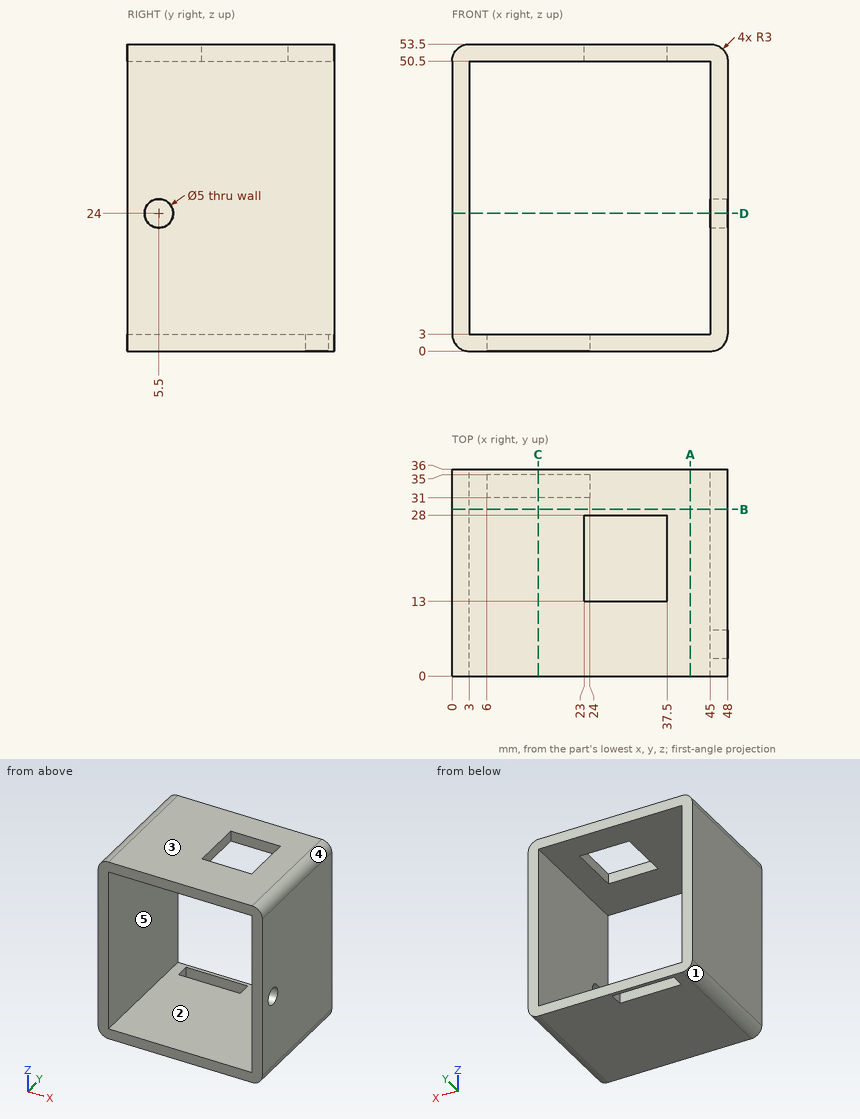
Drawing for the job (mm, zero at the part's lowest x, y, z). A direction names the side the tool comes from. Round coordinates to 2 decimals unless told otherwise and drop trailing zeros. Order: outer loops, then holes, each group sorted by start corner. A loop starts at its lowest first (then second) coordinate and runs counter-clockwise, first axis right, second up. Notation, with made-up numbers: M 56,-37 L 76,-37 A18 cw 76,-7 Z; hole C 1,18 d7. An arc over 180 degrees is marked long. Use one line per item in the form item = value.
Q1. Probe L1, parallel to X at y = 3.5, z = 5; L2, parallel to Y at x = 47.35, z = 24; L3, parallel to Z at x = 34, y = 12.5. List the from-to ranges inside material, lowest first.
Recorded:
L1 = 0 to 3, 45 to 48
L2 = 0 to 3, 8 to 36
L3 = 0 to 3, 50.5 to 53.5
Q2. Saw through at A-A on x = 41.5. Give the cut face in (y, z), then the cut area to 3 significant figures.
Recorded:
outline = M 0,0 L 36,0 L 36,3 L 0,3 Z; M 0,50.5 L 36,50.5 L 36,53.5 L 0,53.5 Z
area = 216 mm^2
Q3. Saw through at D-D on z = 24. Give the cut face in (x, y), then the cut area to 3 significant figures.
Recorded:
outline = M 0,0 L 3,0 L 3,36 L 0,36 Z; M 45,0 L 48,0 L 48,3 L 45,3 Z; M 45,8 L 48,8 L 48,36 L 45,36 Z
area = 201 mm^2
Q4. Saw through at C-C on x = 15. Give the cut face in (y, z), then the cut area to 3 significant figures.
Recorded:
outline = M 0,0 L 31,0 L 31,3 L 0,3 Z; M 0,50.5 L 36,50.5 L 36,53.5 L 0,53.5 Z; M 35,0 L 36,0 L 36,3 L 35,3 Z
area = 204 mm^2
Q5. Two-plate mould, pull along X, no slides. Class the marked faces 3, 4 and 5: +X half, -X half, draft (parallel to the pull), parting line (faces both ways), or undercut.
Recorded:
face_3 = draft
face_4 = +X half
face_5 = undercut
Q6. Saw through at B-B on y = 29. Give the cut face in (x, z).
Recorded:
outline = M 0,3 A3 ccw 3,0 L 45,0 A3 ccw 48,3 L 48,50.5 A3 ccw 45,53.5 L 3,53.5 A3 ccw 0,50.5 Z; hole M 3,3 L 45,3 L 45,50.5 L 3,50.5 Z
Q7. Which spindle directions (+Z, -Z, +X, -X, +Y, -Y) get a long thin tool onto all of the face, cutting with end or side? Do the marked faces 1 and 2. Say none if no direction does.
Recorded:
face_1 = -Z, -X, +Y, -Y
face_2 = +Y, -Y
Q8. Flat gauge pins, fed straight in: P1, Ø2.5, axis at y = 33.5, z = 1.5, coming from the -X side; P2, Ø0.9, axis at y = 33, z = 1.5, coming from the +X side; P3, Ø0.9, axis at y = 23.5, z = 52.5, coming from the +X side. Where does each tip first touch, or does it go through?
Recorded:
P1 = 0.01
P2 = 47.81
P3 = 47.57
